```python
from build123d import *

# Parameters (mm, degrees)
CUT_EXTRUDE1_DEPTH = 79.89866919


with BuildPart() as part:
    # Sketch1 → Revolve1 (revolve)
    with BuildSketch(Plane.XY, mode=Mode.PRIVATE) as revolve1_sk:
        Polygon((-17.5, 5), (17.5, 5), (17.5, 20), (2.5, 20), (2.5, 40), (17.5, 40), (17.5, 50), (-17.5, 50), (-17.5, 40), (-2.5, 40), (-2.5, 20), (-17.5, 20), align=None)
    revolve(revolve1_sk.sketch.rotate(Axis((-17.5, 0, 0), (1, 0, 0)), 90), axis=Axis((-17.5, 0, 0), (1, 0, 0)))

    # Sketch2 → Cut-Extrude1 (cut, through all)
    with BuildSketch(Plane(origin=(17.5, 0, 0), x_dir=(0, 0, -1), z_dir=(1, 0, 0))):
        with BuildLine():
            Line((2.5, -4.330127019), (2.5, -7.830127019))
            Line((2.5, -7.830127019), (-2.5, -7.830127019))
            Line((-2.5, -7.830127019), (-2.5, -4.330127019))
            ThreePointArc((-2.5, -4.330127019), (0, -5), (2.5, -4.330127019))
        make_face()
    extrude(amount=-CUT_EXTRUDE1_DEPTH, mode=Mode.SUBTRACT)


solid = part.part
```
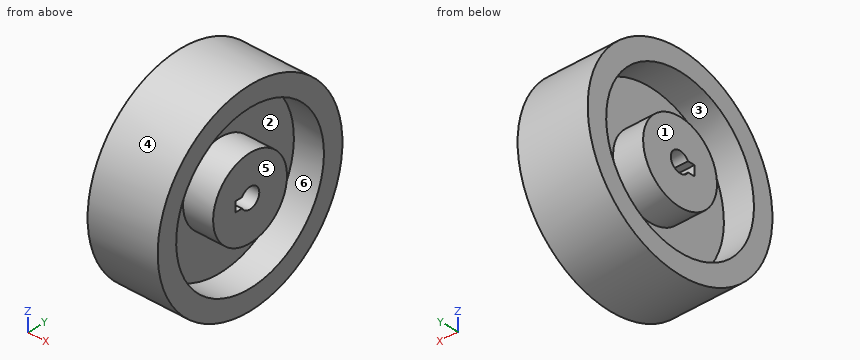
Geometry check sheet. Reference: the model listing, model coordinates, mm. Face numbers are marked on the shaded views. A direction names the side the tool comes from. Coordinates: 2 decimals unless noted, no trailing zeros. Order: outer loops, then holes, each group sorted by start corner. A loop starts at its lowest first (then second) coordinate and runs counter-clockwise, first axis right, second up. Notation, with made-up numbers: M 15,-12 L 52,-12 A11 cw 52,-1 Z; hole C 3.25,32.5 d11. An arc over 180 degrees is marked long. Answer as a JSON object with one key per item and string values.
Q1. Cross-section at B-B on y = 0. Record the cut outline in (x, z), and give its area (3 significant figures).
Results are:
{"outline": "M -17.5,-50 L 17.5,-50 L 17.5,-40 L 2.5,-40 L 2.5,-20 L 17.5,-20 L 17.5,-5 L -17.5,-5 L -17.5,-20 L -2.5,-20 L -2.5,-40 L -17.5,-40 Z; M -17.5,5 L 17.5,5 L 17.5,20 L 2.5,20 L 2.5,40 L 17.5,40 L 17.5,50 L -17.5,50 L -17.5,40 L -2.5,40 L -2.5,20 L -17.5,20 Z", "area": "1,950 mm²"}
Q2. Release check for a two-part mould opening along Y. For the marked faces 4, 5 and 6 record: released by +Y, released by -Y, zero draft, split by the parting line, or undercut.
Results are:
{"face 4": "split by the parting line", "face 5": "zero draft", "face 6": "undercut"}
Q3. Depth check by flat-ended pin: pin 1 Ø5.5 at (x, z) = (2, 0.5) entering from +Y; pin 2 Ø3 at (x, y) = (0, -5.5) entering from +Z; pin 3 Ø6 at (y, z) = (27, -19) entering from -X. Enter the tip coordinate at first touch or a pass-through.
Results are:
{"pin 1": "stops at y = 50", "pin 2": "stops at z = 49.84", "pin 3": "stops at x = -2.5"}
Q4. Scan lines: line 1 (Y direction, x = 13, z = 0); line 2 (Z direction, x = 10.5, y = 0.5); line 3 (Z direction, x = 11.5, y = 2.5). Record each from-to range of solid material in increasing order.
Results are:
{"line 1": "y = -50 to -40, -20 to -7.83, 5 to 20, 40 to 50", "line 2": "z = -50 to -40, -19.99 to -4.97, 4.97 to 19.99, 40 to 50", "line 3": "z = -49.94 to -39.92, -19.84 to -4.33, 4.33 to 19.84, 39.92 to 49.94"}
Q5. Tool access check on the marked faces 1, 2 and 3. Record the directions out of +Z, -Z, +X, -X, +Y, -Y that give a thin tool (end or side, any length) a straight path to the whole face; none if there is none.
Results are:
{"face 1": "+Z, -Z, -X, +Y, -Y", "face 2": "+X", "face 3": "-X"}
Q6. Cross-section at A-A on x = 4. Record the cut outline in (y, z).
Results are:
{"outline": "C 0,0 d100; C 0,0 d40; hole C 0,0 d80; hole M -7.83,-2.5 L -4.33,-2.5 A5 ccw long -4.33,2.5 L -7.83,2.5 Z"}
Q7. Cross-section at D-D on y = -14.5. Record the cut outline in (x, z).
Results are:
{"outline": "M -17.5,-47.85 L 17.5,-47.85 L 17.5,-37.28 L 2.5,-37.28 L 2.5,-13.77 L 17.5,-13.77 L 17.5,13.77 L 2.5,13.77 L 2.5,37.28 L 17.5,37.28 L 17.5,47.85 L -17.5,47.85 L -17.5,37.28 L -2.5,37.28 L -2.5,13.77 L -17.5,13.77 L -17.5,-13.77 L -2.5,-13.77 L -2.5,-37.28 L -17.5,-37.28 Z"}
Q8. Cross-section at C-C on z = 0. Record the cut outline in (x, y), and give its area (3 significant figures).
Results are:
{"outline": "M -17.5,-50 L 17.5,-50 L 17.5,-40 L 2.5,-40 L 2.5,-20 L 17.5,-20 L 17.5,-7.83 L -17.5,-7.83 L -17.5,-20 L -2.5,-20 L -2.5,-40 L -17.5,-40 Z; M -17.5,5 L 17.5,5 L 17.5,20 L 2.5,20 L 2.5,40 L 17.5,40 L 17.5,50 L -17.5,50 L -17.5,40 L -2.5,40 L -2.5,20 L -17.5,20 Z", "area": "1,850 mm²"}
